Could you check a few things on this drawing? It's one solid part, dimensions in mm from its lowest x, y, z. A direction names the side the tool comes from. Coordinates: 2 decimals unless noted, no trailing zeros. Order: outer loops, then holes, each group sorted by start corner. A loop starts at its lowest first (then second) coordinate and runs counter-clockwise, first axis right, second up. Notation, with made-up numbers: M -33,79 L -3,79 A20 ccw -3,108 Z; hole C -3,40.25 d1. An arc over 180 degrees is marked long. Answer as CSV lines item,"result". Start each with the question number.
1. Will these pins go through, and if not, where does the flat tip stop? pin 1 (12 mm diameter, centred on x = 33, y = 32, fed in from +Z) (3 decimals); pin 2 (8 mm diameter, centred on x = 7, z = 10, fed in from -Y); pin 3 (4 mm diameter, centred on y = 6, z = 9.5, fed in from +X).
2. On a 3-axis mill with a long thin cutter (end or side, diameter ignored), from which of +Z, -Z, +X, -X, +Y, -Y can I reach the whole of each face in a straight line? I mean the marked faces 1 and 2. Say none if no direction works.
3. If we section it at C-C (y = 7): List the corners of the cut face in (x, z) for me (1 decimal), plus the area to 3 significant figures.
4. If we section it at B-B (x = 10): List the corners of the cut face in (y, z) for me (1 decimal), plus the area to 3 significant figures.
5. I need wall thicknesses on line 1 along Y through (x, z) = (17, 1.5); line 2 along Y through (x, z) = (43, 8.5) (1 decimal); line 3 along X through (y, z) = (34, 6.75) (1 decimal). Which ranges of each line are inside material? Lowest first, please. Write a range as from..to.
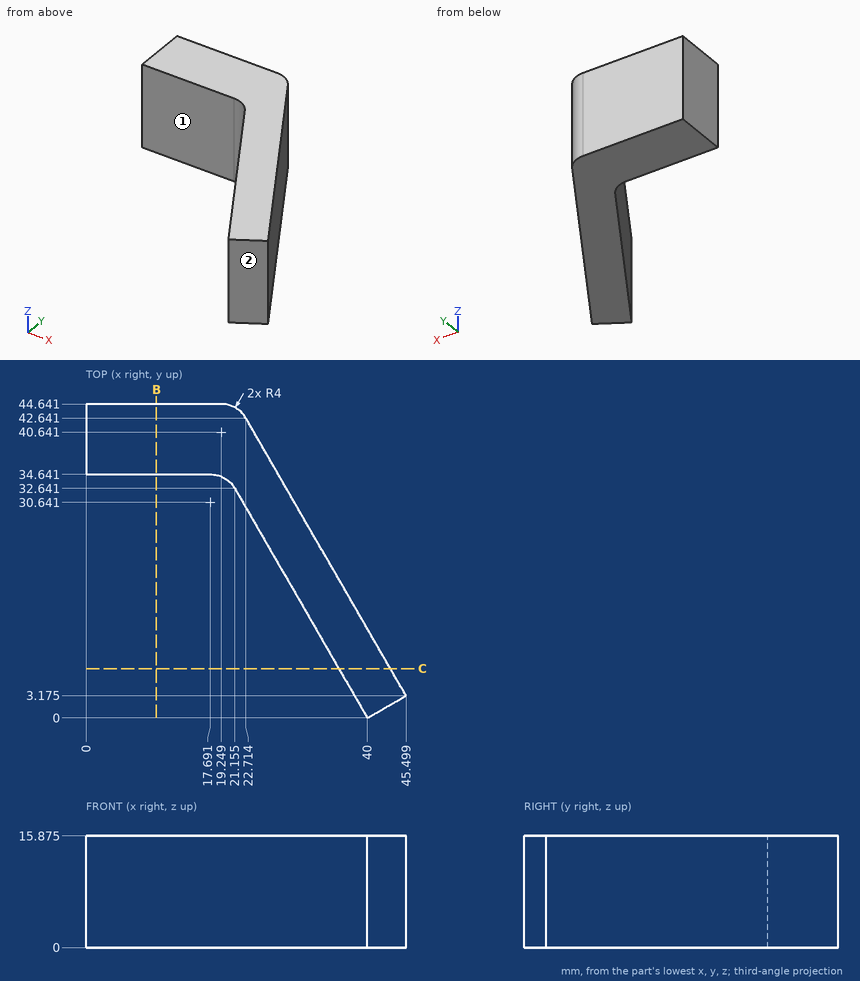
Solved:
1,pin 1,"z = 15.875"
1,pin 2,"y = 34.64"
1,pin 3,"x = 45.02"
2,face 1,"+Z, -Z, -X, -Y"
2,face 2,"+Z, -Z, +X, -Y"
3,outline,"M 36,0 L 43.3,0 L 43.3,15.9 L 36,15.9 Z"
3,area,"116 mm²"
4,outline,"M 34.6,0 L 44.6,0 L 44.6,15.9 L 34.6,15.9 Z"
4,area,"159 mm²"
5,line 1,"34.64..44.64"
5,line 2,"1.7..7.5"
5,line 3,"19.9..27.7"
